Can you work these out from the model? Positions are in its coordinate system, mm. A direction names the side the tool comes from. Coordinates: 2 decimals unless noted, no trailing zeros. Order: outer loops, then holes, each group sorted by start corner. A loop starts at its lowest first (then second) coordinate and runs counter-clockwise, first axis right, second up. Notation, with made-up numbers: (82, 14.5) -> (102, 14.5) arc R9 cw to (102, 24.5) -> close; hole circle Ø11 at (83, -13). An arc over 180 degrees is marked (long way). Write item = value, one per line. Start each with the question number.
from build123d import *

# Parameters (mm, degrees)
F1_DEPTH = 6.604
F2_R     = 13.335
F3_DEPTH = 4.7498
F4_R     = 2.286
F5_DEPTH = 6.604


with BuildPart() as f1:
    # F0 (on Top) → F1 (new body)
    with BuildSketch(Plane.XY):
        with BuildLine():
            ThreePointArc((-1.712611, -3.474329), (0, -3.8735), (1.712611, -3.474329))
            Line((1.712611, -3.474329), (0.898419, -1.822599))
            ThreePointArc((0.898419, -1.822599), (0, -2.032), (-0.898419, -1.822599))
            Line((-0.898419, -1.822599), (-1.712611, -3.474329))
        make_face()
        with BuildLine():
            Line((-1.129208, 1.689353), (-2.152552, 3.220329))
            ThreePointArc((-2.152552, 3.220329), (-3.354549, 1.93675), (-3.865163, 0.254))
            Line((-3.865163, 0.254), (-2.027627, 0.133246))
            ThreePointArc((-2.027627, 0.133246), (-1.759764, 1.016), (-1.129208, 1.689353))
        make_face()
        with BuildLine():
            Line((2.027627, 0.133246), (3.865163, 0.254))
            ThreePointArc((3.865163, 0.254), (3.354549, 1.93675), (2.152552, 3.220329))
            Line((2.152552, 3.220329), (1.129208, 1.689353))
            ThreePointArc((1.129208, 1.689353), (1.759764, 1.016), (2.027627, 0.133246))
        make_face()
        with BuildLine():
            ThreePointArc((2.027627, -0.133246), (2.030906, -0.066659), (2.032, 0))
            ThreePointArc((2.032, 0), (2.030906, 0.066659), (2.027627, 0.133246))
            ThreePointArc((2.027627, 0.133246), (1.759764, 1.016), (1.129208, 1.689353))
            ThreePointArc((1.129208, 1.689353), (1.016, 1.759764), (0.898419, 1.822599))
            ThreePointArc((0.898419, 1.822599), (0, 2.032), (-0.898419, 1.822599))
            ThreePointArc((-0.898419, 1.822599), (-1.016, 1.759764), (-1.129208, 1.689353))
            ThreePointArc((-1.129208, 1.689353), (-1.759764, 1.016), (-2.027627, 0.133246))
            ThreePointArc((-2.027627, 0.133246), (-2.032, 0), (-2.027627, -0.133246))
            ThreePointArc((-2.027627, -0.133246), (-1.759764, -1.016), (-1.129208, -1.689353))
            ThreePointArc((-1.129208, -1.689353), (-1.016, -1.759764), (-0.898419, -1.822599))
            ThreePointArc((-0.898419, -1.822599), (0, -2.032), (0.898419, -1.822599))
            ThreePointArc((0.898419, -1.822599), (1.016, -1.759764), (1.129208, -1.689353))
            ThreePointArc((1.129208, -1.689353), (1.759764, -1.016), (2.027627, -0.133246))
        make_face()
    extrude(amount=F1_DEPTH)

    # F2 (on face) → F3 (join)
    with BuildSketch(Plane.XY.offset(6.604)):
        Circle(F2_R)
    extrude(amount=F3_DEPTH)

    # F4 (on face) → F5 (cut, through all)
    with BuildSketch(Plane(origin=(0, 0, 0), x_dir=(1, 0, 0), z_dir=(0, 0, -1))):
        Circle(F4_R)
    extrude(amount=-F5_DEPTH, mode=Mode.SUBTRACT)


solid = f1.part
(1) Imagine slicing it at B-B (x = 0). Write out the boundary of the cut face in (y, z) (1 decimal), plus the area to 3 significant figures.
(2) For P1, Ø1.5, axis at y = 0, z = 4, coming from the -X side; P2, Ø4, axis at y = -9.5, z = 6, coming from the -X side; P3, Ø4, axis at y = -4.5, z = 8.5, coming from the -X side; P4, Ø5, axis at y = -0.5, z = 8, coming from the -X side (3 decimals), each with a flat end and sliding along its axis, tell me the tip position at first contact or that it passes through.
(3) If I drill on L1, parallel to Z at x = -3, y = -3.5; L2, parallel to X at y = 1, z = 5.75; L3, parallel to Y at x = 0.25, z = 7, over which ranges is the centre line in solid material (lowest first)? Write a range as from..to.
(4) Imagine slicing it at A-A (z = 2.75). Write out the boundary of the cut face in (x, y).
(5) For faces 5 (the face through (-3.34, 1.96, 3.26)), 6 (the face through (0, 0, 6.604)), 7 (the face through (-3.084, 0.203, 3.256)), 8 (the face through (-0.025, -3.873, 3.256)), which set-ups out of +Z, -Z, +X, -X, +Y, -Y let a thin tool reach every point of the face, with its end or its side?
(6) Imagine slicing it at D-D (z = 9.25). Write out the boundary of the cut face in (x, y) (3 decimals), plus the area to 3 significant figures.
(7) Imagine slicing it at C-C (y = 4.75). Write out the boundary of the cut face in (x, z).
(8) Thinking about a two-plate mould opening in Y: for faces 1 (the face through (0, -3, 0)), 2 (the face through (1.367, -2.772, 3.256)), 3 (the face through (1.72, 2.57, 3.26)), 4 (the face through (3.06, 0.2, 3.26)), which applies, +Y half, -Y half, draft (parallel to the pull), parting line (faces both ways), or undercut?
Result set:
q1.outline = (-13.3, 6.6) -> (-3.9, 6.6) -> (-3.9, 0) -> (-2.3, 0) -> (-2.3, 6.6) -> (13.3, 6.6) -> (13.3, 11.4) -> (-13.3, 11.4) -> close
q1.area = 137 mm2
q2.P1 = -3.87
q2.P2 = -10.96
q2.P3 = -13.1
q2.P4 = -13.335
q3.L1 = 6.6..11.35
q3.L2 = -3.74..-2.06, 2.06..3.74
q3.L3 = -13.33..13.33
q4.outline = (-3.87, 0.25) -> (-2.28, 0.15) arc R2.29 cw to (-1.27, 1.9) -> (-2.15, 3.22) arc R3.87 ccw to start; (-1.71, -3.47) arc R3.87 ccw to (1.71, -3.47) -> (1.01, -2.05) arc R2.29 cw to (-1.01, -2.05) -> close; (1.27, 1.9) arc R2.29 cw to (2.28, 0.15) -> (3.87, 0.25) arc R3.87 ccw to (2.15, 3.22) -> close
q5.face_5 = -Z, -X, +Y
q5.face_6 = -Z
q5.face_7 = -Z, -X, -Y
q5.face_8 = -Z, -Y
q6.outline = circle Ø26.67 at (0, 0)
q6.area = 559 mm2
q7.outline = (-12.46, 6.6) -> (12.46, 6.6) -> (12.46, 11.35) -> (-12.46, 11.35) -> close
q8.face_1 = draft
q8.face_2 = undercut
q8.face_3 = +Y half
q8.face_4 = -Y half
